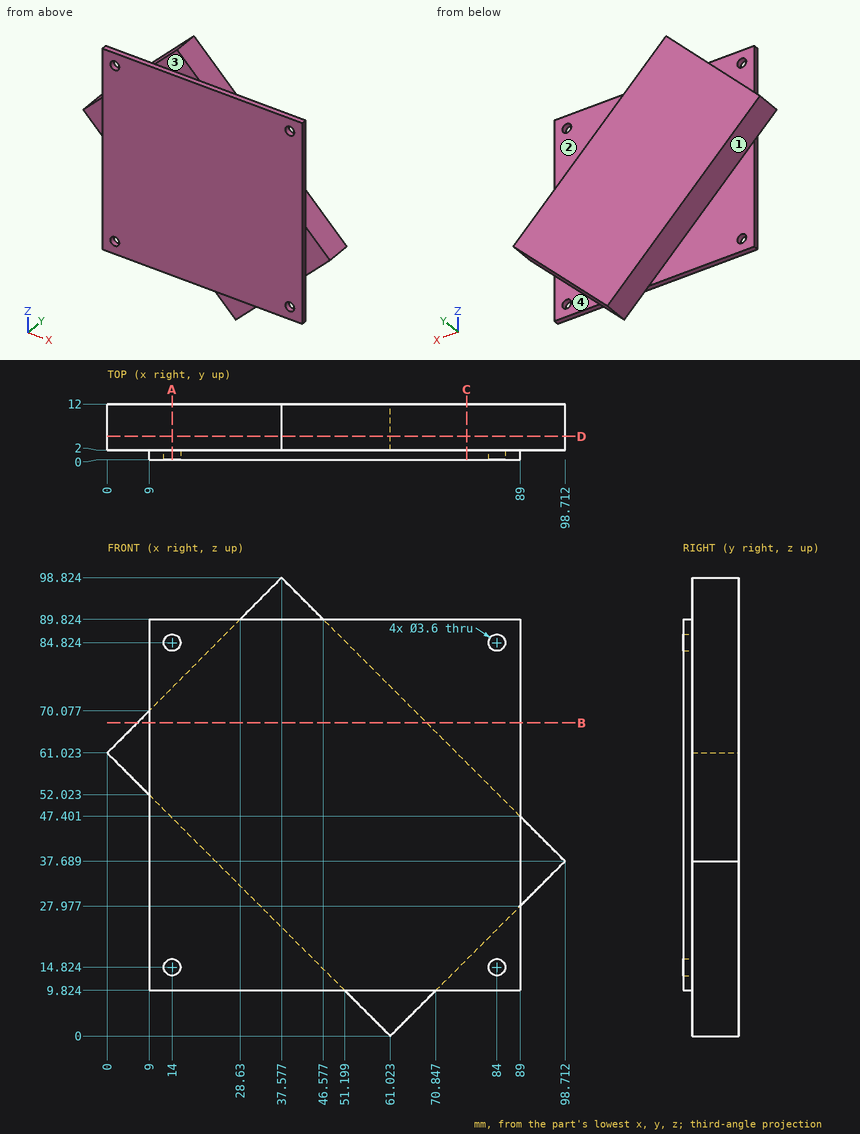
For this review, use the dimensioned drawing (mm, ordinates from the lowest corner) and the shaded views. A direction names the side the tool comes from. Coordinates: 2 decimals unless noted, no trailing zeros. Order: outer loops, then holes, each group sorted by start corner. A loop starts at its lowest first (then second) coordinate and runs counter-clockwise, first axis right, second up. Notation, with made-up numbers: (65.5, 63.25) - (124.5, 63.25) arc R17 ccw to (124.5, 78.25) - close; hole circle Ø7 at (79, 87.25). An arc over 180 degrees is marked (long way). Answer in a Markdown table with one row per item.
(1) Consider section C-C on x = 77.5. State the section outline as (y, z) points, plus the area to 3 significant figures.
Checked values:
| item | result |
|---|---|
| outline | (0, 9.82) - (2, 9.82) - (2, 16.48) - (12, 16.48) - (12, 58.9) - (2, 58.9) - (2, 89.82) - (0, 89.82) - close |
| area | 584 mm^2 |
(2) For the marked faces 1, 2, 3 and 4, list the 3-axis set-ups (+Z, -Z, +X, -X, +Y, -Y) from which the entire face can be reached by the end or side of a thin tool; tool diameter is ignored.
Checked values:
| item | result |
|---|---|
| face 1 | -Z, -X, +Y |
| face 2 | +Z, +X, +Y |
| face 3 | +Z, +X, -X, -Y |
| face 4 | -Z, +X, +Y |
(3) Consider section A-A on x = 14. State the section outline as (y, z) points.
Checked values:
| item | result |
|---|---|
| outline | (0, 9.82) - (2, 9.82) - (2, 13.02) - (0, 13.02) - close; (0, 16.62) - (2, 16.62) - (2, 47.02) - (12, 47.02) - (12, 75.11) - (2, 75.11) - (2, 83.02) - (0, 83.02) - close; (0, 86.62) - (2, 86.62) - (2, 89.82) - (0, 89.82) - close |
(4) Consider section B-B on z = 67.5. State the section outline as (x, y) points.
Checked values:
| item | result |
|---|---|
| outline | (6.44, 2) - (9, 2) - (9, 0) - (89, 0) - (89, 2) - (68.9, 2) - (68.9, 12) - (6.44, 12) - close |
(5) Consider section D-D on y = 5. State the section outline as (x, z) points.
Checked values:
| item | result |
|---|---|
| outline | (0, 61.02) - (61.02, 0) - (98.71, 37.69) - (37.58, 98.82) - close |
(6) Wall thickness on line 1 along Z through (x, y) = (14, 0.9); line 2 along Y through (x, z) = (34, 17); line 3 along Z through (x, y) = (58, 1.5): over which ranges is each line inside the solid? List them lowest first. Write a range as from..to.
Checked values:
| item | result |
|---|---|
| line 1 | 9.82..13.02, 16.62..83.02, 86.62..89.82 |
| line 2 | 0..2 |
| line 3 | 9.82..89.82 |
(7) Clearance check with flat-ended pins moving along their axes: pin 1 (2 mm diameter, centred on y = 0.5, z = 58.5, fed in from +X); pin 2 (1 mm diameter, centred on y = 6, z = 23, fed in from -X) (1 decimal); pin 3 (2 mm diameter, centred on y = 7.5, z = 79.5, fed in from +X); pin 4 (15.5 mm diameter, centred on x = 14.5, z = 78, fed in from +Y). State where each tip first meets the part, or that it passes through.
Checked values:
| item | result |
|---|---|
| pin 1 | x = 89 |
| pin 2 | x = 37.5 |
| pin 3 | x = 57.9 |
| pin 4 | y = 12 |
